Input: part model. Units: mm. Frame: model coordinates. A direction names the side the tool comes from. Give positions to 0.01 mm unless a question says otherwise; leave off trailing zeros. Loops run counter-clockwise (first coordinate to the right, second up) from the corner with the lowest first, then second, coordinate; pieces in that order, holes last. Notation, with made-up numbers: (-38.75, -39.5) - (-11.75, -39.5) arc R15 cw to (-11.75, -34.5) - close; hole circle Ø6 at (-12, 46.25). An arc over 180 degrees is marked (long way). One line per item, written item: value.
from build123d import *

# Parameters (mm, degrees)
ESBO_O1_W                = 20
ESBO_O1_H                = 10
RESSALTO_EXTRUS_O1_DEPTH = 75
FURO1_D                  = 6.35
FURO1_DEPTH              = 14.916024102
FURO1_CBORE_D            = 9.52
FURO1_CBORE_DEPTH        = 6.35
RESSALTO_EXTRUS_O2_DEPTH = 20


with BuildPart() as part:
    # Esboço1 → Ressalto-extrusão1 (new body)
    with BuildSketch(Plane.XY):
        Rectangle(ESBO_O1_W, ESBO_O1_H)
    extrude(amount=RESSALTO_EXTRUS_O1_DEPTH)

    # Furo1
    with Locations(Plane(origin=(0, 5, 0), x_dir=(1, 0, 0), z_dir=(0, 1, 0))):
        with Locations((0, -6.5)):
            CounterBoreHole(FURO1_D / 2, FURO1_CBORE_D / 2, FURO1_CBORE_DEPTH, depth=FURO1_DEPTH)

    # Esboço4 → Ressalto-extrusão2 (add)
    with BuildSketch(Plane.XY.offset(75)):
        with BuildLine():
            Line((-10, 5), (10, 5))
            ThreePointArc((10, 5), (0, 7.087121525), (-10, 5))
        make_face()
    extrude(amount=-RESSALTO_EXTRUS_O2_DEPTH)


solid = part.part
Item 1: Section B-B, the plane x = 0. Output: boundary loops of the cut face in (y, z) (3 decimals).
Verdict:
outline: (-5, 0) - (5, 0) - (5, 1.74) - (-1.35, 1.74) - (-1.35, 3.325) - (-5, 3.325) - close; (-5, 9.675) - (-1.35, 9.675) - (-1.35, 11.26) - (5, 11.26) - (5, 55) - (7.087, 55) - (7.087, 75) - (-5, 75) - close
Item 2: Draft query along X for faces 1 (the face through (-1.5, -3.2, 9.3)), 2 (the face through (-10, 0, 37)), 3 (the face through (10, 0, 37)). Return one class per face: pulls with the +X half, pulls with the -X half, needs draft (parallel to the pull), parting line crosses it, or undercut.
Verdict:
face 1: undercut
face 2: pulls with the -X half
face 3: pulls with the +X half
Item 3: Material intervals for L1, parallel to Z at x = 0, y = -3.55 (3 decimals); L2, parallel to Z at x = 0, y = 0.5; L3, parallel to Y at x = 1.25, z = 53.5, sorted ascending.
Verdict:
L1: z = 0 to 3.325, 9.675 to 75
L2: z = 0 to 1.74, 11.26 to 75
L3: y = -5 to 5
Item 4: Access query for faces 4 (the face through (0, 5, 27)), 5 (the face through (0, 1, 75)), 6 (the face through (1, -1.35, 10)). Directions: +Z, -Z, +X, -X, +Y, -Y. A direction counts if a zero-diameter tool reaches every point of the face in a straight line with its end or side. Return the directions, or none.
Verdict:
face 4: -Z, +X, -X, +Y
face 5: +Z, +X, -X, +Y, -Y
face 6: +Y
Item 5: Section D-D, the plane x = 4. Output: boundary loops of the cut face in (y, z), and give its area (3 significant figures).
Verdict:
outline: (-5, 0) - (5, 0) - (5, 3.92) - (-1.35, 3.92) - (-1.35, 9.08) - (5, 9.08) - (5, 55) - (6.77, 55) - (6.77, 75) - (-5, 75) - close
area: 753 mm^2
Item 6: Pin query (flat end, axial travel): P1, Ø12, axis at x = 2, z = 16.5, coming from the +Y side; P2, Ø1, axis at x = 1, y = 6.5, coming from the -Z side. Return the tip coordinate at first contact, or that it passes through.
Verdict:
P1: stops at y = 5
P2: stops at z = 55
Item 7: Section C-C, the plane y = 1.5. Output: boundary loops of the cut face in (x, z), and give its area (3 significant figures).
Verdict:
outline: (-10, 0) - (10, 0) - (10, 75) - (-10, 75) - close; hole circle Ø9.52 at (0, 6.5)
area: 1,430 mm^2
Item 8: Section A-A, the plane z = 6.5. Output: boundary loops of the cut face in (x, y) (3 decimals), and give its area (3 significant figures).
Verdict:
outline: (-10, -5) - (-3.175, -5) - (-3.175, -1.35) - (-4.76, -1.35) - (-4.76, 5) - (-10, 5) - close; (3.175, -5) - (10, -5) - (10, 5) - (4.76, 5) - (4.76, -1.35) - (3.175, -1.35) - close
area: 116 mm^2
